from build123d import *

# Parameters (mm, degrees)
SKETCH1_W               = 20
SKETCH1_H               = 20
BOSS_EXTRUDE1_DEPTH     = 38
SKETCH2_R               = 1
CUT_EXTRUDE1_DEPTH      = 2.5
SKETCH3_R               = 8
BOSS_EXTRUDE2_DEPTH     = 1.5
SKETCH4_R               = 2
BOSS_EXTRUDE3_DEPTH     = 10
CUT_EXTRUDE2_DEPTH      = 11
CUT_EXTRUDE2_DEPTH_BACK = 11
CHAMFER1_SIZE           = 0.25
FILLET1_R               = 1
SKETCH6_W               = 10
SKETCH6_H               = 2.5
BOSS_EXTRUDE4_DEPTH     = 12


with BuildPart() as part:
    # Sketch1 → Boss-Extrude1 (new body)
    with BuildSketch(Plane(origin=(0, 0, 0), x_dir=(1, 0, 0), z_dir=(0, 1, 0))):
        Rectangle(SKETCH1_W, SKETCH1_H)
    extrude(amount=-BOSS_EXTRUDE1_DEPTH)

    # Sketch2 → Cut-Extrude1 (cut)
    with BuildSketch(Plane(origin=(0, 0, 0), x_dir=(1, 0, 0), z_dir=(0, 1, 0))):
        with Locations((-7.7, 7.7)):
            Circle(SKETCH2_R)
        with Locations((7.7, 7.7)):
            Circle(SKETCH2_R)
        with Locations((7.7, -7.7)):
            Circle(SKETCH2_R)
        with Locations((-7.7, -7.7)):
            Circle(SKETCH2_R)
    extrude(amount=-CUT_EXTRUDE1_DEPTH, mode=Mode.SUBTRACT)

    # Sketch3 → Boss-Extrude2 (add)
    with BuildSketch(Plane(origin=(0, 0, 0), x_dir=(1, 0, 0), z_dir=(0, 1, 0))):
        Circle(SKETCH3_R)
    extrude(amount=BOSS_EXTRUDE2_DEPTH)

    # Sketch4 → Boss-Extrude3 (add)
    with BuildSketch(Plane(origin=(0, 0, 0), x_dir=(1, 0, 0), z_dir=(0, 1, 0))):
        Circle(SKETCH4_R)
    extrude(amount=BOSS_EXTRUDE3_DEPTH)

    # Sketch5 → Cut-Extrude2 (cut, two sides)
    with BuildSketch(Plane.XY) as cut_extrude2_sk:
        Polygon((2, 10), (1.5, 10), (1.5, 3), (2, 2.5), align=None)
    extrude(amount=CUT_EXTRUDE2_DEPTH, mode=Mode.SUBTRACT)
    extrude(cut_extrude2_sk.sketch, amount=-CUT_EXTRUDE2_DEPTH_BACK, mode=Mode.SUBTRACT)

    # Chamfer1
    chamfer1_edges = [part.edges().sort_by_distance(p)[0] for p in [
        (-2, 10, 0),
    ]]
    chamfer(chamfer1_edges, length=CHAMFER1_SIZE)

    # Fillet1
    fillet1_edges = [part.edges().sort_by_distance(p)[0] for p in [
        (10, -38, 0),
        (0, -38, -10),
        (-10, -38, 0),
        (0, -38, 10),
        (-10, -19, -10),
        (10, -19, -10),
        (10, -19, 10),
        (-10, -19, 10),
    ]]
    fillet(fillet1_edges, radius=FILLET1_R)

    # Sketch6 → Boss-Extrude4 (add)
    with BuildSketch(Plane(origin=(0, 0, 0), x_dir=(0, 0, -1), z_dir=(1, 0, 0))):
        with Locations((0, -33)):
            Rectangle(SKETCH6_W, SKETCH6_H)
    extrude(amount=BOSS_EXTRUDE4_DEPTH)


solid = part.part
Work out the finished part from the listing and answer in its coordinate system (mm). A direction names the side the tool comes from. Give positions to 0.01 mm unless a question says otherwise; leave off trailing zeros. Loops run counter-clockwise (first coordinate to the right, second up) from the corner with the lowest first, then second, coordinate; pieces in that order, holes last. Notation, with made-up numbers: (57, -16) -> (71, -16) arc R25 cw to (71, 9) -> close; hole circle Ø5 at (-0.75, -33.5). An arc over 180 degrees is marked (long way). Use a Markdown table: item, result. Add a question column.
1. Section A-A on z = 0 is taken. Determine the outline of the cut face in (x, y), and give its area (3 significant figures).
2. Section C-C on z = 3.75 is taken. Determine the outline of the cut face in (x, y), and give its area (3 significant figures).
3. Flat-ended cylindrical pins translate along their axes: pin 1 Ø1.6 at (x, z) = (10.5, 0) entering from -Y; pin 2 Ø5 at (y, z) = (-30, -6) entering from +X; pin 3 Ø0.6 at (x, y) = (11, -32.5) entering from -Z; pin 4 Ø0.8 at (y, z) = (7, 0.5) entering from +X. Find the tip coordinate at first contact, or state that the pin passes through.
4. Find the intervals of material crossed by probe 1 along Z at (x, y) = (-7.7, -1.05); probe 2 along Y at (x, z) = (4.75, -1.25), in increasing order.
5. Section B-B on x = 0 is taken. Determine the outline of the cut face in (y, z).
6. For faces 1 (the flat face through (11, -33, -5)), 2 (the cylindrical face through (-9.715, -18.759, -9.699)), 3 (the flat face through (-5, 0, -7)), 4 (the flat face through (1.5, 7, 0)), determine the directions among +Z, -Z, +X, -X, +Y, -Y from which every point of the face is accessible in a straight line to the end or side of a thin tool.
7. Determine the mould class of faces 5 (the flat face through (-10, -18, 0)), 6 (the cylindrical face through (8.624, -1.232, -7.317)), 7 (the cylindrical face through (9.699, -18.759, -9.715)), 8 (the cylindrical face through (-6.776, -1.232, 8.083)) for opening direction Z: released by +Z, released by -Z, zero draft, split by the parting line, or undercut.
Results below:
| question | item | result |
|---|---|---|
| 1 | outline | (-10, -37) arc R1 ccw to (-9, -38) -> (9, -38) arc R1 ccw to (10, -37) -> (10, -34.25) -> (12, -34.25) -> (12, -31.75) -> (10, -31.75) -> (10, 0) -> (8, 0) -> (8, 1.5) -> (2, 1.5) -> (2, 2.5) -> (1.5, 3) -> (1.5, 10) -> (-1.75, 10) -> (-2, 9.75) -> (-2, 1.5) -> (-8, 1.5) -> (-8, 0) -> (-10, 0) -> close |
| 1 | area | 819 mm^2 |
| 2 | outline | (-10, -37) arc R1 ccw to (-9, -38) -> (9, -38) arc R1 ccw to (10, -37) -> (10, -34.25) -> (12, -34.25) -> (12, -31.75) -> (10, -31.75) -> (10, 0) -> (7.07, 0) -> (7.07, 1.5) -> (-7.07, 1.5) -> (-7.07, 0) -> (-10, 0) -> close |
| 2 | area | 786 mm^2 |
| 3 | pin 1 | stops at y = -37.71 |
| 3 | pin 2 | stops at x = 12 |
| 3 | pin 3 | stops at z = -5 |
| 3 | pin 4 | stops at x = 1.5 |
| 4 | probe 1 | z = -10 to -8.7, -6.7 to 6.7, 8.7 to 10 |
| 4 | probe 2 | y = -38 to 1.5 |
| 5 | outline | (-38, -9) arc R1 ccw to (-37, -10) -> (0, -10) -> (0, -8) -> (1.5, -8) -> (1.5, -2) -> (9.75, -2) -> (10, -1.75) -> (10, 1.75) -> (9.75, 2) -> (1.5, 2) -> (1.5, 8) -> (0, 8) -> (0, 10) -> (-37, 10) arc R1 ccw to (-38, 9) -> close |
| 6 | face 1 | -Z, +X, +Y, -Y |
| 6 | face 2 | -Z, -X, +Y, -Y |
| 6 | face 3 | +Y |
| 6 | face 4 | +Z, -Z, +X, +Y |
| 7 | face 5 | zero draft |
| 7 | face 6 | undercut |
| 7 | face 7 | released by -Z |
| 7 | face 8 | undercut |
